Autodesk Inventor part; units mm, degrees
ref_plane "YZ Plane" through (0, 0, 0) normal (1, 0, 0) x (0, 1, 0)
ref_plane "XZ Plane" through (0, 0, 0) normal (0, 1, 0) x (-1, 0, 0)
ref_plane "XY Plane" through (0, 0, 0) normal (0, 0, 1) x (1, 0, 0)
sketch "Esboço1" plane through (0, 0, 0) normal (0, 0, 1) x (1, 0, 0)
  line L0 (-119, 0) -> (119, 0) construction
  line L1 (0, -159) -> (0, 79) construction
  line L2 (-5, 45) -> (5, 45)
  line L3 (5, 45) -> (5, -45)
  line L4 (5, -45) -> (-5, -45)
  line L5 (-5, -45) -> (-5, 45)
  circle A0 centre (0, -40) radius 5
  circle A1 centre (0, 40) radius 5
  circle A2 centre (0, 42) radius 3
  line L6 (-5, 39) -> (5, 39)
  line L7 (5, 39) -> (5, -35)
  line L8 (5, -35) -> (-5, -35)
  line L9 (-5, -35) -> (-5, 39)
  circle A3 centre (0, -40) radius 85
  point P0 (0, 0)
  point P1 (5, 39)
  point P2 (-5, -35)
  dimension "d0" = 10
  dimension "d2" = 85
  dimension "d3" = 90
  dimension "d4" = 6
  dimension "d20" = 170
extrude "Extrusão1" add sketch "Esboço1" against normal blind 6 contours L2 A3 L5 | A3 L3 A1 | A2 L6 A1 | A1 L6 A2 | A2 | L2 L3 A3 | A1 L5 A3 | L3 L6 A1 | A1 L6 L5 | L6 A1 | L3 L8 L5 L6 A1 | L3 A0 L8 | L8 A0 L5 | A0 | L3 L4 A0 | A0 L4 L5
extrude "Extrusão2" cut sketch "Esboço1" along normal blind 0.5 from surface at -6 contours L6 A1 | L3 L8 L5 L6 A1 | L3 A0 L8 | L8 A0 L5 | A0 | L3 L4 A0 | A0 L4 L5
extrude "Extrusão3" cut sketch "Esboço1" along normal blind 2.5 from surface at -5.5 contours L6 A1 | L3 L8 L5 L6 A1
hole "Furo1" at (0, -40, 0) direction (0, 0, -1) diameter 4.5 end through all counterbore diameter 6.5 counterbore depth 3.5
fillet "Arredondamento1" radius 0.5 8 edges at (-5, 39, -4.5) (5, 39, -4.5) (-5, 45, -3) (5, 45, -3) (-5, -35, -4.25) (-5, -45, -2.75) (5, -45, -2.75) (5, -35, -4.25)
properties part number "VEJ-00-015" material "Fenolite OR"
Input: part model. Units: mm. Frame: model coordinates. A direction names the side the tool comes from. Round coordinates to 2 decimals unless told otherwise and drop trailing zeros. Loops run counter-clockwise (first coordinate to the right, second up) from the corner with the lowest first, then second, coordinate; pieces in that order, holes last.
1) Section query B-B on x = 0. Return the cut outline in (y, z).
Ans:
outline: (-45, -5.5) - (-42.25, -5.5) - (-42.25, -3.5) - (-43.25, -3.5) - (-43.25, 0) - (-45, 0) - close; (-37.75, -5.5) - (-35, -5.5) - (-35, -3) - (39, -3) - (39, -6) - (45, -6) - (45, 0) - (-36.75, 0) - (-36.75, -3.5) - (-37.75, -3.5) - close
2) Section query A-A on z = -4.25. Return the cut outline in (x, y), plus the area to 3 significant figures.
Ans:
outline: (-5, -44.5) arc R0.5 ccw to (-4.5, -45) - (4.5, -45) arc R0.5 ccw to (5, -44.5) - (5, -35.5) arc R0.5 ccw to (4.5, -35) - (-4.5, -35) arc R0.5 ccw to (-5, -35.5) - close; (-5, 39.5) arc R0.5 ccw to (-4.5, 39) - (4.5, 39) arc R0.5 ccw to (5, 39.5) - (5, 44.5) arc R0.5 ccw to (4.5, 45) - (-4.5, 45) arc R0.5 ccw to (-5, 44.5) - close; hole circle Ø4.5 at (0, -40)
area: 144 mm2
3) Section query C-C on y = -40. Return the cut outline in (x, z).
Ans:
outline: (-5, -5.5) - (-2.25, -5.5) - (-2.25, -3.5) - (-3.25, -3.5) - (-3.25, 0) - (-5, 0) - close; (2.25, -5.5) - (5, -5.5) - (5, 0) - (3.25, 0) - (3.25, -3.5) - (2.25, -3.5) - close
4) Material intervals for line 1 (Y direction, x = 0, z = -4.4); line 2 (Y direction, x = -3.5, z = -3.7); line 3 (X direction, y = -40, z = -1.75), sorted ascending.
Ans:
line 1: y = -45 to -42.25, -37.75 to -35, 39 to 45
line 2: y = -45 to -35, 39 to 45
line 3: x = -5 to -3.25, 3.25 to 5
5) Set-up query: faces 5 (the flat face through (0, 39, -5)), 6 (the flat face through (0, 45, -3)), 7 (the flat face through (-1.2, -37.7, -5.5)). Return all of +Z, -Z, +X, -X, +Y, -Y with unobstructed straight access to the full face (end or side cutting, diameter ignored); none if empty.
Ans:
face 5: -Z, +X, -X
face 6: +Z, -Z, +X, -X, +Y
face 7: -Z, +X, -X, -Y
6) Pull-direction query (X, two-part tool) for faces 1 (the flat face through (5, 1, -2)), 2 (the flat face through (0, 42, -6)), 3 (the cylindrical face through (1.245, -43.002, -1.774)), 4 (the cylindrical face through (-0.099, -37.752, -4.514)); classes: released by +X, released by -X, zero draft, split by the parting line, or undercut.
Ans:
face 1: released by +X
face 2: zero draft
face 3: undercut
face 4: undercut
7) Pin query (flat end, axial travel): pin 1 (1 mm diameter, centred on x = 3, y = 29, fed in from -Z); pin 2 (5 mm diameter, centred on x = 0, y = -40, fed in from +Z); pin 3 (5 mm diameter, centred on x = 0, y = -40, fed in from -Z). Return the tip coordinate at first contact, or that it passes through.
Ans:
pin 1: stops at z = -3
pin 2: stops at z = -3.5
pin 3: stops at z = -5.5
